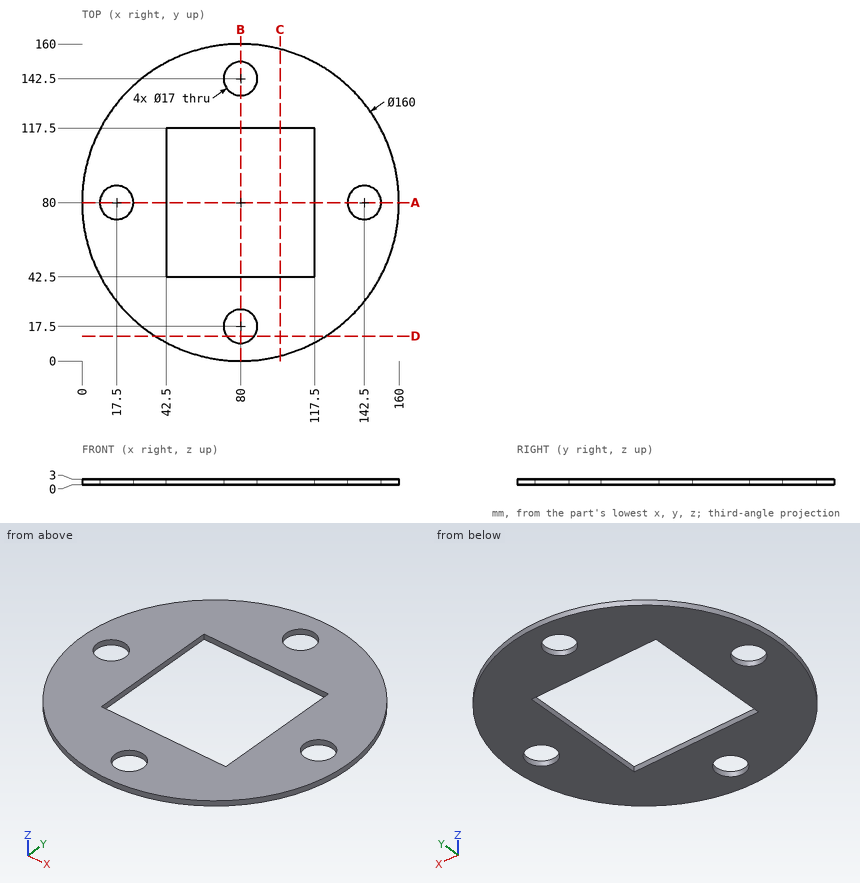
Geometry: see drawing. Coordinates: mm, zero at the bounding-box minimum. Give positions to 0.01 mm unless a question says otherwise; leave off trailing zeros. Order: outer loops, then holes, each group sorted by start corner. A loop starts at its lowest first (then second) coordinate and runs counter-clockwise, first axis right, second up. Notation, with made-up numbers: (11.5, 44.5) - (54.5, 44.5) arc R28 ccw to (54.5, 64.5) - close; hole circle Ø5 at (29, -11.75). An arc over 180 degrees is marked (long way). Use CSV: the item, a comma, the result in double quotes.
1. Material intervals for line 1 along Y through (x, z) = (80, 2.1); line 2 along X through (y, z) = (86.5, 1.75); line 3 along Y through (x, z) = (86, 1.05), sorted ascending. Write a range as from..to.
Answers below:
line 1,"0..9, 26..42.5, 117.5..134, 151..160"
line 2,"0.26..12.02, 22.98..42.5, 117.5..137.02, 147.98..159.74"
line 3,"0.23..11.48, 23.52..42.5, 117.5..136.48, 148.52..159.77"
2. Contact query for flat-ended pins moving along their axis: pin 1 (0.9 mm diameter, centred on x = 91.5, z = 1.5, fed in from -Y); pin 2 (0.9 mm diameter, centred on y = 71, z = 1.5, fed in from -X); pin 3 (1.5 mm diameter, centred on y = 131.5, z = 0.5, fed in from -X). Output: stop coordinate, or through.
Answers below:
pin 1,"y = 0.77"
pin 2,"x = 0.46"
pin 3,"x = 18.16"
3. Section query A-A (y = 80). Output: boundary loops of the cut face in (x, z).
Answers below:
outline,"(0, 0) - (9, 0) - (9, 3) - (0, 3) - close; (26, 0) - (42.5, 0) - (42.5, 3) - (26, 3) - close; (117.5, 0) - (134, 0) - (134, 3) - (117.5, 3) - close; (151, 0) - (160, 0) - (160, 3) - (151, 3) - close"
4. Section query C-C (x = 100). Output: boundary loops of the cut face in (y, z), plus the area to 3 significant figures.
Answers below:
outline,"(2.54, 0) - (42.5, 0) - (42.5, 3) - (2.54, 3) - close; (117.5, 0) - (157.46, 0) - (157.46, 3) - (117.5, 3) - close"
area,"240 mm2"
5. Section query D-D (y = 12.5). Output: boundary loops of the cut face in (x, z).
Answers below:
outline,"(37.06, 0) - (73.13, 0) - (73.13, 3) - (37.06, 3) - close; (86.87, 0) - (122.94, 0) - (122.94, 3) - (86.87, 3) - close"
